The model under review builds one solid part; all positions refer to its coordinate system, in mm. A direction names the side the tool comes from. Give positions to 0.01 mm unless a question says otherwise; leave off trailing zeros. Write each loop counter-clockwise with the first axis right and the second up, starting at its lowest first coordinate (ties: lowest second). Pieces come first, ordered by that corner, then holes. Notation, with made-up numbers: M 45.25,73.25 L 98.25,73.25 A26 cw 98.25,100.25 Z; hole C -32.5,-20.75 d9. An arc over 180 degrees is marked long. Write each question's results on one line, items separated by ' | '. Start each with the question number.
Autodesk Inventor part; units mm, degrees
ref_plane "YZ Plane" through (0, 0, 0) normal (1, 0, 0) x (0, 1, 0)
ref_plane "XZ Plane" through (0, 0, 0) normal (0, 1, 0) x (-1, 0, 0)
ref_plane "XY Plane" through (0, 0, 0) normal (0, 0, 1) x (1, 0, 0)
sketch "Sketch1" plane through (0, 0, 0) normal (0, 0, 1) x (1, 0, 0)
  circle A0 centre (0, 0) radius 14.25
  circle A1 centre (0, 0) radius 20
  line L0 (0, 20) -> (10, 20)
  line L1 (10, 20) -> (10, 17.3205)
  line L2 (0, 20) -> (0, 20)
  line L3 (0, 20) -> (-10, 20)
  line L4 (-10, 20) -> (-10, 17.3205)
  point P0 (-20, 0)
  point P1 (20, 0)
  dimension "d0" = 28.5
  dimension "d1" = 40
  dimension "d25" = 10
  dimension "d31" = 10
  dimension "d32" = 0
extrude "Extrusion1" add sketch "Sketch1" along normal blind 10
ref_plane "Work Plane1" through (0, 0, -10) normal (0, 0, 1) x (1, 0, 0)
mirror "Mirror1" about plane through (0, 0, -10) normal (0, 0, 1) of "Extrusion1"
sketch "Sketch2" plane through (0, 0, -30) normal (0, 0, -1) x (-1, 0, 0)
  circle A0 centre (0, 0) radius 14.25
  circle A1 centre (0, 0) radius 20
  dimension "d11" = 40
extrude "Extrusion2" add sketch "Sketch2" along normal blind 3 contours A0 | A1
sketch "Sketch3" plane through (0, 0, -30) normal (0, 0, 1) x (1, 0, 0)
  circle A0 centre (0, 0) radius 3.15
  dimension "d14" = 6.3
extrude "Extrusion3" cut sketch "Sketch3" against normal blind 1
sketch "Sketch4" plane through (0, 0, -31) normal (0, 0, 1) x (1, 0, 0)
  circle A0 centre (0, 0) radius 3.15
  line L0 (0, 0) -> (0, -1.6)
  line L1 (0, -1.6) -> (-2.7134, -1.6)
  line L2 (0, -1.6) -> (2.7134, -1.6)
  dimension "d17" = 6.3
  dimension "d18" = 1.6
extrude "Extrusion4" cut sketch "Sketch4" against normal through all contours A0 L2 L1 picked at (-0.0447, 1.5505)
sketch "Sketch6" plane through (-7.5, 20, -22) normal (0, 1, 0) x (1, 0, 0)
  line L0 (17.5, 8) -> (17.5, 8)
  line L1 (17.5, -22) -> (17.5, -32)
  line L2 (-2.5, 8) -> (17.5, 8)
  line L3 (17.5, 8) -> (17.5, -32)
  line L4 (17.5, -32) -> (-2.5, -32)
  line L5 (-2.5, -32) -> (-2.5, 8)
  point P0 (7.5, -22)
extrude "Extrusion6" add sketch "Sketch6" along normal blind 5
sketch "Sketch7" plane through (-7.5, 25, -22) normal (0, 1, 0) x (1, 0, 0)
  line L0 (21.75, -32) -> (-6.75, -32)
  line L1 (7.5, -32) -> (7.5, 8)
  line L2 (10.65, 8) -> (4.35, 8)
  circle A0 centre (7.5, -12) radius 4.25
  point P0 (7.5, -22)
  dimension "d28" = 8.5
extrude "Extrusion7" cut sketch "Sketch7" against normal up to next
chamfer "Chamfer1" distance 5 angle 45 1 edges at (-14.25, 0, -20)
equation "\"d4\" = d25"
equation "\"BendRadius\" = Thickness"
equation "\"BendReliefWidth\" = Thickness"
equation "\"BendReliefDepth\" = 0.5 * Thickness"
equation "\"CornerReliefSize\" = 4 * Thickness"
equation "\"MinimumRemnant\" = 2 * Thickness"
equation "\"TransitionRadius\" = BendRadius"
equation "\"JacobiRadiusSize\" = BendRadius"
equation "\"GapSize\" = Thickness"
properties part number "baseRotor1"
(1) Add section D-D (z = 2). State the section outline as (x, y) points.
(2) Machinability: for faces 1 (the cylindrical face through (1.69, 2.66, -31.48)), 2 (the flat face through (0, -1.6, -32)), 3 (the flat face through (8, 18, -20)), 4 (the flat face through (-10, 22, -10)), 5 (the conical face through (-3.157, -14.216, -24.687)), which of the approach directions +Z, -Z, +X, -X, +Y, -Y give a long, thin tool a straight path to every point of the face, cutting with its end or side? Answer none if there is none.
(3) Wall thickness on L1, parallel to Y at x = 0, z = -28.8; L2, parallel to Y at x = 0, z = -31.5; L3, parallel to Z at x = -4, y = 19: over which ranges is each line inside the solid? List them lowest first.
(4) Add section C-C (z = -10). State the section outline as (x, y) points.
(5) Add section A-A (y = 0). State the section outline as (x, z) points.
(6) Draft analysis for pull direction X (two halves, no side actions). For faces 6 (the flat face through (-9, 12, 10)), 7 (the flat face through (0, -2, -31)), 8 (the cylindrical face through (0.733, -19.987, 4.93)), 9 (the flat face through (0.2, 3.4, -30)), state which applies: pulls with the +X half, pulls with the -X half, needs draft (parallel to the pull), parting line crosses it, or undercut.
(7) Clearance check with flat-ended pins moving along their axes: P1, Ø5.5, axis at x = 0, y = 0, coming from the +Z side; P2, Ø8.5, axis at y = 21, z = -13, coming from the -X side; P3, Ø2, axis at x = 2.5, z = 2, coming from the -Y side. State where each tip first meets the part, or that it passes through.
(8) Add section B-B (x = 0). Give the number of separate pieces and of enclosed holes in the cut face, then the cut area to 3 significant figures.
Calculated:
1) outline: M -10,17.32 A20 ccw long 10,17.32 L 10,25 L -10,25 Z; hole C 0,0 d28.5
2) face 1: +Z | face 2: +Z, -Z | face 3: +X, -X, -Y | face 4: +Z, -Z, -X, +Y | face 5: none
3) L1: y = -20 to -14.25, 14.25 to 25 | L2: y = -20 to -1.6, 3.15 to 20 | L3: z = -33 to -20, 0 to 10
4) outline: M -10,20 L -4.25,20 L -4.25,25 L -10,25 Z; M 4.25,20 L 10,20 L 10,25 L 4.25,25 Z
5) outline: M -20,-33 L -3.15,-33 L -3.15,-30 L -14.25,-30 L -14.25,-25 L -19.25,-20 L -20,-20 Z; M -20,0 L -14.25,0 L -14.25,10 L -20,10 Z; M 3.15,-33 L 20,-33 L 20,-20 L 19.25,-20 L 14.25,-25 L 14.25,-30 L 3.15,-30 Z; M 14.25,0 L 20,0 L 20,10 L 14.25,10 Z
6) face 6: needs draft | face 7: undercut | face 8: parting line crosses it | face 9: undercut
7) P1: stops at z = -31 | P2: stops at x = -10 | P3: stops at y = -19.94
8) separate pieces: 4 | enclosed holes: 0 | area: 467 mm²
